```python
from build123d import *

# Parameters (mm, degrees)
SKETCH_2_W          = 155
SKETCH_2_H          = 75
EXTRUDE_1_DEPTH     = 15
CUT_EXTRUDE_1_DEPTH = 161.175684796
FILLET_1_R          = 28
EXTRUDE_2_DEPTH     = 100
CHAMFER_1_SIZE      = 95.405683439
CHAMFER_1_SIZE_2    = 5
EXTRUDE_3_DEPTH     = 30
CUT_EXTRUDE_4_REACH = 145.596


with BuildPart() as part:
    # 스케치2 → 보스-돌출1 (new body)
    with BuildSketch(Plane(origin=(0, 0, 0), x_dir=(1, 0, 0), z_dir=(0, 1, 0))):
        Rectangle(SKETCH_2_W, SKETCH_2_H)
    extrude(amount=EXTRUDE_1_DEPTH)

    # 스케치3 → 컷-돌출1 (cut, through all)
    with BuildSketch(Plane(origin=(77.5, 0, 0), x_dir=(0, 0, -1), z_dir=(1, 0, 0))):
        Polygon((37.5, 5), (-37.5, 15), (37.5, 15), align=None)
    extrude(amount=-CUT_EXTRUDE_1_DEPTH, mode=Mode.SUBTRACT)

    # 필렛1
    fillet_1_edges = [part.edges().sort_by_distance(p)[0] for p in [
        (-77.5, 2.5, -37.5),
        (77.5, 2.5, -37.5),
        (77.5, 7.5, 37.5),
        (-77.5, 7.5, 37.5),
    ]]
    fillet(fillet_1_edges, radius=FILLET_1_R)

    # 스케치4 → 보스-돌출2 (add)
    with BuildSketch(Plane.XZ):
        with BuildLine():
            Line((-49.5, 36.5), (49.5, 36.5))
            ThreePointArc((49.5, 36.5), (76.5, 9.5), (49.5, -17.5))
            Line((49.5, -17.5), (-49.5, -17.5))
            ThreePointArc((-49.5, -17.5), (-76.5, 9.5), (-49.5, 36.5))
        make_face()
    extrude(amount=-EXTRUDE_2_DEPTH)

    # 모따기1
    # the kernel refuses this chamfer: 95.405683439, 5 mm, written as the material it takes off along each edge
    with BuildSketch(Plane(origin=(-49.5, 100, 36.5), x_dir=(0, -0.9999979738662977, 0.0020130234223821315), z_dir=(1, 0, 0))) as chamfer_1_piece_1_section:
        Polygon((CHAMFER_1_SIZE * 0.999997973863, CHAMFER_1_SIZE * 0.00201302342237), (-CHAMFER_1_SIZE_2 * 0.00201302342238, CHAMFER_1_SIZE_2 * 0.999997973866), (0, 0), align=None)
    chamfer_1_piece_1 = extrude(amount=99, mode=Mode.PRIVATE)
    chamfer_1_piece_1 = split(chamfer_1_piece_1, bisect_by=Plane(origin=(0, 15.586966884, 41.90225163), z_dir=(0, 0.9912279006826347, -0.13216372009101798)), keep=Keep.TOP, mode=Mode.PRIVATE)
    add(chamfer_1_piece_1, mode=Mode.SUBTRACT)
    with BuildSketch(Plane(origin=(-49.5, 100, 9.5), x_dir=(0, 0, -1), z_dir=(1, 0, 0))) as chamfer_1_piece_2_section:
        Polygon((27, -CHAMFER_1_SIZE), (27 - CHAMFER_1_SIZE_2, 0), (27, 0), align=None)
    chamfer_1_piece_2 = revolve(axis=Axis((-49.5, 100, 9.5), (0, 1, 0)), revolution_arc=180, mode=Mode.PRIVATE)
    chamfer_1_piece_2 = split(chamfer_1_piece_2, bisect_by=Plane(origin=(-74.18479248, 12.010621427, 15.0796607), z_dir=(0, 0.9912279006826347, -0.13216372009101798)), keep=Keep.TOP, mode=Mode.PRIVATE)
    add(chamfer_1_piece_2, mode=Mode.SUBTRACT)
    with BuildSketch(Plane(origin=(49.5, 100, 9.5), x_dir=(0, 0, 1), z_dir=(-1, 0, 0))) as chamfer_1_piece_3_section:
        Polygon((27, -CHAMFER_1_SIZE), (27 - CHAMFER_1_SIZE_2, 0), (27, 0), align=None)
    chamfer_1_piece_3 = revolve(axis=Axis((49.5, 100, 9.5), (0, 1, 0)), revolution_arc=180, mode=Mode.PRIVATE)
    chamfer_1_piece_3 = split(chamfer_1_piece_3, bisect_by=Plane(origin=(74.18479248, 12.010621427, 15.0796607), z_dir=(0, 0.9912279006826347, -0.13216372009101798)), keep=Keep.TOP, mode=Mode.PRIVATE)
    add(chamfer_1_piece_3, mode=Mode.SUBTRACT)
    with BuildSketch(Plane(origin=(49.5, 100, -17.5), x_dir=(0, -0.9999979738662977, -0.0020130234223820955), z_dir=(-1, 0, 0))) as chamfer_1_piece_4_section:
        Polygon((CHAMFER_1_SIZE * 0.999997973863, CHAMFER_1_SIZE * 0.00201302342237), (-CHAMFER_1_SIZE_2 * 0.00201302342238, CHAMFER_1_SIZE_2 * 0.999997973866), (0, 0), align=None)
    chamfer_1_piece_4 = extrude(amount=99, mode=Mode.PRIVATE)
    chamfer_1_piece_4 = split(chamfer_1_piece_4, bisect_by=Plane(origin=(0, 8.9149356, -8.137983001), z_dir=(0, 0.9912279006826347, -0.13216372009101798)), keep=Keep.TOP, mode=Mode.PRIVATE)
    add(chamfer_1_piece_4, mode=Mode.SUBTRACT)

    # 스케치6 → 보스-돌출3 (add)
    with BuildSketch(Plane.XY):
        with BuildLine():
            Line((-51, 67.5), (51, 67.5))
            ThreePointArc((51, 67.5), (56.5, 62), (51, 56.5))
            Line((51, 56.5), (-51, 56.5))
            ThreePointArc((-51, 56.5), (-56.5, 62), (-51, 67.5))
        make_face()
        with BuildLine():
            Line((-51, 40.5), (51, 40.5))
            ThreePointArc((51, 40.5), (56.5, 35), (51, 29.5))
            Line((51, 29.5), (-51, 29.5))
            ThreePointArc((-51, 29.5), (-56.5, 35), (-51, 40.5))
        make_face()
    extrude(amount=-EXTRUDE_3_DEPTH)

    # 컷-돌출4: from a plane face, 145.596 long prism both ways, kept between that surface and its translate by the depth
    cut_extrude_4_start = Plane(origin=(-49.5, 4.594316561, -17.5), z_dir=(0, 0.05233595624294105, -0.998629534754574)) * Box(584.384, 584.384, 292.192, align=(Align.CENTER, Align.CENTER, Align.MIN), mode=Mode.PRIVATE)
    cut_extrude_4_end = Plane(origin=(-49.5, 4.594316561, -17.3), z_dir=(0, 0.05233595624294105, -0.998629534754574)) * Box(584.384, 584.384, 292.192, align=(Align.CENTER, Align.CENTER, Align.MIN), mode=Mode.PRIVATE)
    # 스케치8 → 컷-돌출4 (cut, from a surface)
    with BuildSketch(Plane(origin=(0, 0, -30), x_dir=(-1, 0, 0), z_dir=(0, 0, -1)), mode=Mode.PRIVATE) as cut_extrude_4_sk1:
        with BuildLine():
            Line((-1.75, 90), (1.75, 90))
            ThreePointArc((1.75, 90), (2.75, 89), (1.75, 88))
            Line((1.75, 88), (-1.75, 88))
            ThreePointArc((-1.75, 88), (-2.75, 89), (-1.75, 90))
        make_face()
    cut_extrude_4_tool1 = extrude(cut_extrude_4_sk1.sketch, amount=CUT_EXTRUDE_4_REACH, both=True, mode=Mode.PRIVATE)
    add(((cut_extrude_4_tool1 - cut_extrude_4_start) & cut_extrude_4_end).solids().sort_by_distance((0, 89, -12.976486))[0], mode=Mode.SUBTRACT)


solid = part.part
```
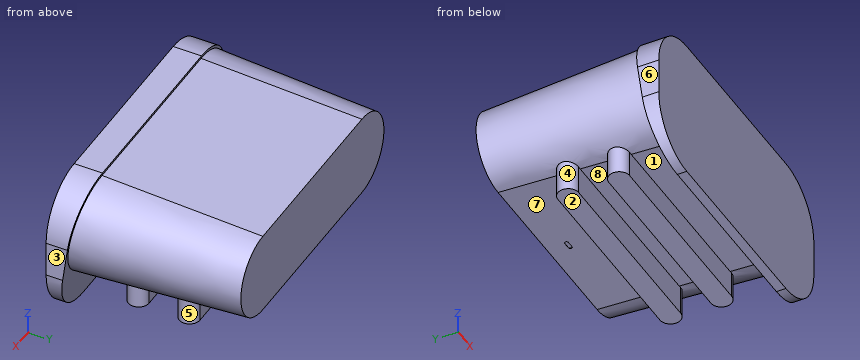
CAD build for the part. Positions are in the model's coordinates, mm. Face numbers are marked on the shaded views. A direction names the side the tool comes from. Coordinates: 2 decimals unless noted, no trailing zeros. Write each loop counter-clockwise with the first axis right and the second up, starting at its lowest first coordinate (ties: lowest second). Pieces come first, ordered by that corner, then holes.
(1) Cut at B-B, the plane y = 35. List the corners of the cut face in (x, z), and give its area (3 significant figures).
(2) Drill centre lines: probe 1 along Y at (x, z) = (-6.5, -24.5); probe 2 along Y at (x, z) = (-47, -34); probe 3 along X at (y, z) = (30, -9). Where is each one in solid material? Low to high.
(3) Cut at A-A, the plane x = 31.5. List the corners of the cut face in (y, z), and give its area (3 significant figures).
(4) Flat gauge pins, fed straight in: pin 1 (7 mm diameter, centred on x = -14, z = -20, fed in from +Y); pin 2 (9 mm diameter, centred on x = -24, y = 60, fed in from -Z); pin 3 (6 mm diameter, centred on y = 14, z = -1, fed in from +X). Where does each tip first touch, or does it go through?
(5) Cut at D-D, the plane y = 46.5. List the corners of the cut face in (x, z).
(6) Cut at C-C, the plane y = 63.5. List the corners of the cut face in (x, z), and give its area (3 significant figures).
(7) 3-axis set-ups, long thin cutter, end or side, ignore diameter. For the marked faces 1, 2, 3, 4 and 5: which of +Z, -Z, +X, -X, +Y, -Y reach the whole face in a straight line?
(8) Two-plate mould, pull along Y, no slides. Class the marked faces 6, 7 and 8: +Y half, -Y half, draft (parallel to the pull), parting line (faces both ways), or undercut.
Geometry says:
1. outline: (-56.5, -30) - (56.5, -30) - (56.5, -14.92) arc R25.41 ccw to (49.5, 34.91) - (-49.5, 34.91) arc R25.41 ccw to (-56.5, -14.92) - close
1. area: 8,660 mm2
2. probe 1: y = 0 to 6.73, 29.5 to 40.5, 56.5 to 67.5
2. probe 2: y = 0 to 5.47
2. probe 3: x = -67.29 to 67.29
3. outline: (0, -37.5) - (5, -37.5) - (7.69, -17.34) - (29.5, -16.19) - (29.5, -30) - (40.5, -30) - (40.5, -15.62) - (56.5, -14.78) - (56.5, -30) - (67.5, -30) - (67.5, -14.2) - (100, -12.5) - (100, 31.5) - (14.8, 35.97) - (15, 37.5) - (0, 37.5) - close
3. area: 5,390 mm2
4. pin 1: stops at y = 67.5
4. pin 2: stops at z = -30
4. pin 3: stops at x = 74.94
5. outline: (-49.5, -15.3) - (49.5, -15.3) arc R24.8 ccw to (49.5, 34.3) - (-49.5, 34.3) arc R24.8 ccw to start
6. outline: (-56.29, -30) - (56.29, -30) - (56.29, -13.43) arc R23.91 ccw to (49.5, 33.41) - (-49.5, 33.41) arc R23.91 ccw to (-56.29, -13.43) - close
6. area: 8,290 mm2
7. face 1: -Z, +X, -X
7. face 2: -Z, +X, -X, +Y
7. face 3: +Z, -Z, +X, +Y, -Y
7. face 4: -Z, -X
7. face 5: -Z, +X
8. face 6: draft
8. face 7: +Y half
8. face 8: undercut
